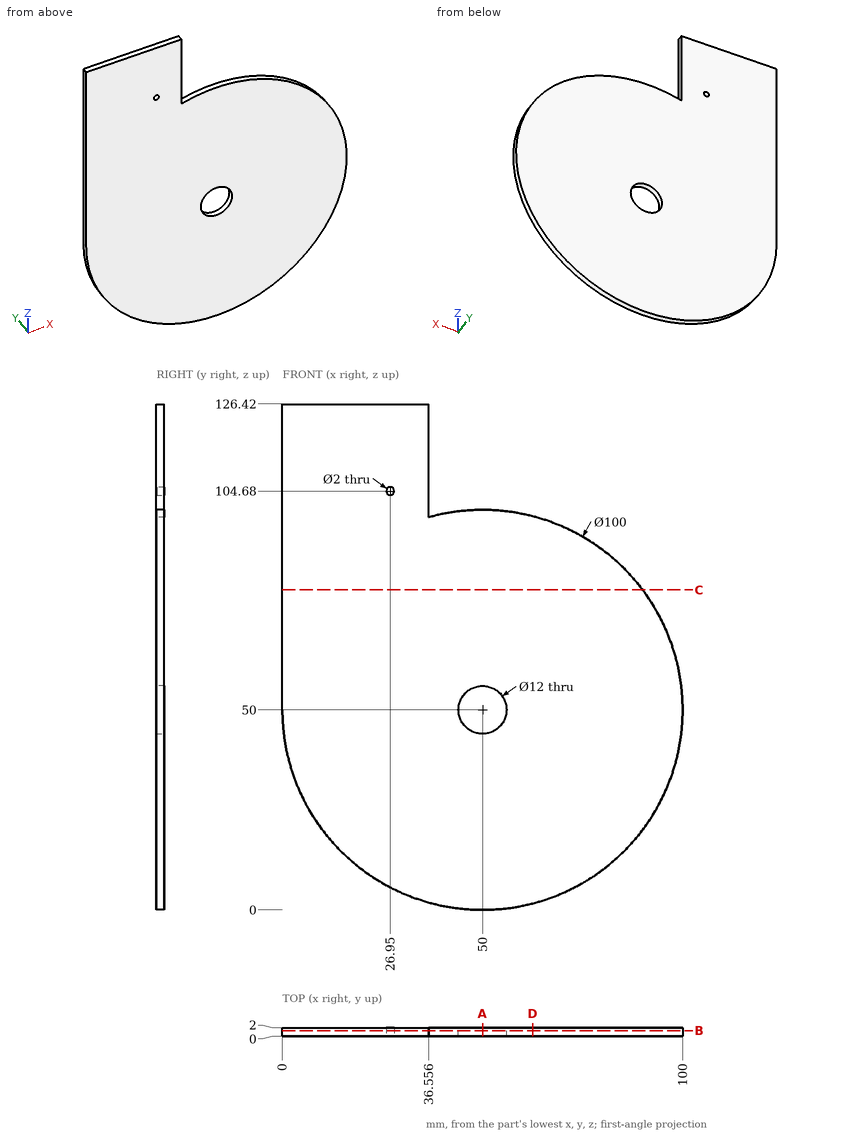
Study the drawing (mm; zero at the part's minimum x, y, z) and answer. Give positions to 0.01 mm unless a question says otherwise; leave off trailing zeros. Loops run counter-clockwise (first coordinate to the right, second up) from the corner with the lowest first, then second, coordinate; pieces in that order, holes last. Notation, with made-up numbers: (-2.5, 41.25) - (23.5, 41.25) arc R21 ccw to (23.5, 61.25) - close; hole circle Ø4 at (44, 81.5). An arc over 180 degrees is marked (long way). Answer in a Markdown table with one row per item. Add a question column.
Q1. Consider line 1 along X through (y, z) = (0.15, 110) (1 decimal); line 2 along X through (y, z) = (0.7, 50); line 3 along Z through (x, y) = (52, 1.05). Determine where each line is inside the solid, lowest interval first.
Q2. The part is cut by section A-A (x = 50). Determine the outline of the cut face in (y, z), and give its area (3 significant figures).
Q3. The part is cut by section C-C (z = 80). Determine the outline of the cut face in (x, y), and give its area (3 significant figures).
Q4. The part is cut by section B-B (y = 1.35). State how many separate pieces and enclosed holes the cut face has, and give its area (3 significant figures).
Q5. Each of these flat-tipped pins is pushed along its axis until it touches: P1, Ø1.6, axis at x = 26.95, z = 104.68, coming from the -Y side; P2, Ø1, axis at y = 1, z = 118.5, coming from the +X side. Where does it stop, or does it pass through?
Q6. The part is cut by section D-D (x = 62.5). Determine the outline of the cut face in (y, z).
Solution:
| question | item | result |
|---|---|---|
| 1 | line 1 | x = 0 to 36.6 |
| 1 | line 2 | x = 0 to 44, 56 to 100 |
| 1 | line 3 | z = 0.04 to 44.34, 55.66 to 99.96 |
| 2 | outline | (0, 0) - (2, 0) - (2, 44) - (0, 44) - close; (0, 56) - (2, 56) - (2, 100) - (0, 100) - close |
| 2 | area | 176 mm² |
| 3 | outline | (0, 0) - (90, 0) - (90, 2) - (0, 2) - close |
| 3 | area | 180 mm² |
| 4 | separate pieces | 1 |
| 4 | enclosed holes | 2 |
| 4 | area | 9,230 mm² |
| 5 | P1 | passes through |
| 5 | P2 | stops at x = 36.56 |
| 6 | outline | (0, 1.59) - (2, 1.59) - (2, 98.41) - (0, 98.41) - close |
